```python
from build123d import *

# Parameters (mm, degrees)
BOSS_EXTRUDE1_DEPTH = 13.3
SKETCH2_R           = 0.65
BOSS_EXTRUDE2_DEPTH = 1
FILLET1_R           = 0.3
FILLET2_R           = 0.3


with BuildPart() as part:
    # Sketch1 → Boss-Extrude1 (new body)
    with BuildSketch(Plane(origin=(0, 0, 0), x_dir=(1, 0, 0), z_dir=(0, 1, 0))):
        Polygon((7.25, 0), (5.126524164, 5.126524164), (0, 7.25), (-5.126524164, 5.126524164), (-7.25, 0), (-5.126524164, -5.126524164), (0, -7.25), (5.126524164, -5.126524164), align=None)
    extrude(amount=BOSS_EXTRUDE1_DEPTH)

    # Sketch2 → Boss-Extrude2 (add)
    with BuildSketch(Plane(origin=(0, 13.3, 0), x_dir=(1, 0, 0), z_dir=(0, 1, 0))):
        with Locations(Location((0, 0, 0), (0, 0, 270))):  # turned: the seam where the file's is
            Circle(SKETCH2_R)
    extrude(amount=BOSS_EXTRUDE2_DEPTH)

    # Fillet1
    fillet1_edges = [part.edges().sort_by_distance(p)[0] for p in [
        (5.126524164, 6.65, 5.126524164),
        (0, 6.65, 7.25),
        (-5.126524164, 6.65, 5.126524164),
        (-7.25, 6.65, 0),
        (-5.126524164, 6.65, -5.126524164),
        (0, 6.65, -7.25),
        (5.126524164, 6.65, -5.126524164),
        (7.25, 6.65, 0),
    ]]
    fillet(fillet1_edges, radius=FILLET1_R)

    # Fillet2
    fillet2_edges = [part.edges().sort_by_distance(p)[0] for p in [
        (0, 13.3, -0.65),
        (-2.563262082, 13.3, 6.188262082),
        (-6.188262082, 13.3, 2.563262082),
        (6.188262082, 13.3, 2.563262082),
        (6.188262082, 13.3, -2.563262082),
        (2.563262082, 13.3, -6.188262082),
        (-2.563262082, 13.3, -6.188262082),
        (-6.188262082, 13.3, -2.563262082),
        (2.563262082, 13.3, 6.188262082),
        (0, 13.3, 7.22528234),
        (5.109046139, 13.3, 5.109046139),
        (7.22528234, 13.3, 0),
        (5.109046139, 13.3, -5.109046139),
        (0, 13.3, -7.22528234),
        (-5.109046139, 13.3, -5.109046139),
        (-7.22528234, 13.3, 0),
        (-5.109046139, 13.3, 5.109046139),
    ]]
    fillet(fillet2_edges, radius=FILLET2_R)


solid = part.part
```
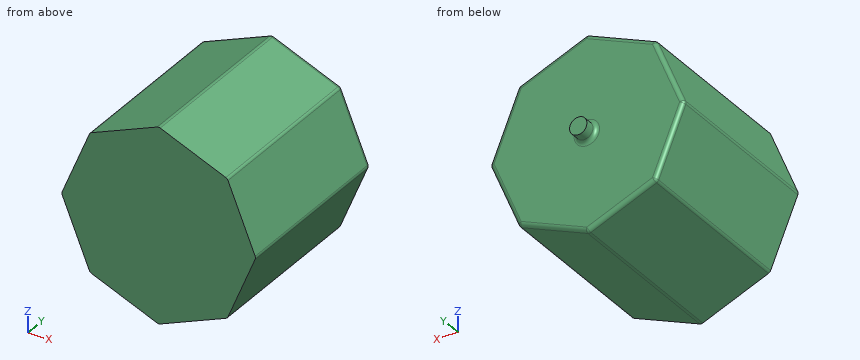
Design review of the part built by this model. Coordinates are the model's own, in mm. Round coordinates to 2 decimals unless told otherwise and drop trailing zeros. Order: outer loops, then holes, each group sorted by start corner. A loop starts at its lowest first (then second) coordinate and runs counter-clockwise, first axis right, second up. Notation, with made-up numbers: (-8.5, 29) - (-3.5, 29) arc R15 ccw to (-3.5, 56) - close; hole circle Ø6 at (-19, 25.5). An arc over 180 degrees is marked (long way). One line per question, with ' | ' between items.
Item 1: Wall thickness on line 1 (Y direction, x = 1, z = -6); line 2 (Z direction, x = 5, y = 10.25); line 3 (Z direction, x = -1.75, y = 3.75): over which ranges is each line inside the solid? List them lowest first. Write a range as [from, to].
Checks:
line 1: [0, 13.3] | line 2: [-5.18, 5.18] | line 3: [-6.53, 6.53]
Item 2: Take a section at A-A, the plane y = 1.5. Write out the cut boundary in (x, z), then the cut area to 3 significant figures.
Checks:
outline: (-7.2, -0.11) - (-5.17, -5.01) arc R0.3 ccw to (-5.01, -5.17) - (-0.11, -7.2) arc R0.3 ccw to (0.11, -7.2) - (5.01, -5.17) arc R0.3 ccw to (5.17, -5.01) - (7.2, -0.11) arc R0.3 ccw to (7.2, 0.11) - (5.17, 5.01) arc R0.3 ccw to (5.01, 5.17) - (0.11, 7.2) arc R0.3 ccw to (-0.11, 7.2) - (-5.01, 5.17) arc R0.3 ccw to (-5.17, 5.01) - (-7.2, 0.11) arc R0.3 ccw to start | area: 149 mm²
Item 3: For P1, Ø6, axis at y = 9.5, z = -5.5, coming from the -X side; P2, Ø5, axis at x = 5, z = 1, coming from the +Y side; P3, Ø5, axis at x = 5.5, y = 11, coming from the +Z side, all flat-tipped, find the tip position at first contact; note any pin that passes through.
Checks:
P1: x = -6.21 | P2: y = 13.3 | P3: z = 6.01
